Read the model definition and answer for the solid it produces. Units are mm, in the model's axes. A direction names the side the tool comes from. Round coordinates to 2 decimals unless told otherwise and drop trailing zeros. Order: outer loops, then holes, each group sorted by start corner. A loop starts at its lowest first (then second) coordinate and runs counter-clockwise, first axis right, second up. Notation, with made-up numbers: (-38, 1) - (-4, 1) arc R3 cw to (-4, 5) - close; hole circle Ø2 at (50.5, 24.25). An arc over 180 degrees is marked (long way). One line per question, with ' | ' between items. Start each with the question number.
1) Flat-ended cylindrical pins translate along their axes: pin 1 (2 mm diameter, centred on x = 90, z = 0, fed in from -Y); pin 2 (2 mm diameter, centred on y = 15, z = 0, fed in from +X); pin 3 (1.8 mm diameter, centred on x = -150, z = 0, fed in from +Y); pin 4 (11 mm diameter, centred on x = 59, y = 25, fed in from +Z). Find the tip coordinate at first contact, or state that the pin passes through.
2) The mould has two halves that part along Y. Classify faces 3 (the flat face through (-2, 1, -3)), 4 (the flat face through (75.622, -20.278, 1.521)), 5 (the flat face through (-2, 61.188, 0)): pulls with the +Y half, pulls with the -Y half, needs draft (parallel to the pull), parting line crosses it, or undercut.
3) For faces 1 (the flat face through (-2, -61.188, 0)), 2 (the flat face through (63.8, -22.9, 1.5)), determine the directions among +Z, -Z, +X, -X, +Y, -Y from which every point of the face is accessible in a straight line to the end or side of a thin tool.
4) The part is cut by section A-A, the plane y = -34. Give the vertices of the cut face in (x, z).
5) Straight lines are drawn through the part: line 1 (Y direction, x = -146.05, z = 0); line 2 (Z direction, x = -120, y = -57); line 3 (Y direction, x = 104, z = 0.2). For each, find the intervals that lie inside material, in ascending order. Write a range as from..to.
from build123d import *

# Parameters (mm, degrees)
SKETCH_1_W                     = 306
SKETCH_1_H                     = 122.375397488
EXTRUDE_1_DEPTH                = 3
M3X0_5_2_D                     = 2.5
M3X0_5_2_DEPTH                 = 8.5
M3X0_5_2_CBORE_D               = 3
M3X0_5_2_CBORE_DEPTH           = 6
M3X0_5_2_TIP                   = 0.751075774
M3X0_5_2_ON_FACE_2_D           = 2.5
M3X0_5_2_ON_FACE_2_DEPTH       = 8.5
M3X0_5_2_ON_FACE_2_CBORE_D     = 3
M3X0_5_2_ON_FACE_2_CBORE_DEPTH = 6
M3X0_5_2_ON_FACE_2_TIP         = 0.751075774
PATTERN_LINEAR_1_COUNT         = 11
PATTERN_LINEAR_1_PITCH         = 30
CUT_EXTRUDE_1_DEPTH            = 3


# Read off the part's stored shape, not the designer's step: M3x0.5 ねじ穴1
with BuildPart() as part:
    # ｽｹｯﾁ1 → ﾎﾞｽ - 押し出し1 (new, symmetric)
    with BuildSketch(Plane.XY):
        Rectangle(SKETCH_1_W, SKETCH_1_H)
    extrude(amount=EXTRUDE_1_DEPTH, both=True)

    # M3x0.5 ねじ穴1 outline → M3x0.5 ねじ穴1 (revolve, cut)
    with BuildSketch(Plane(origin=(-150, 0, 0), x_dir=(1, 0, 0), z_dir=(0, 0, 1))):
        Polygon((1.25, -52.687698744), (0, -51.93662297), (0, -61.187698744), (1.5, -61.187698744), (1.5, -55.187698744), (1.25, -55.187698744), align=None)
        Polygon((0, 61.187698744), (0, 51.93662297), (1.25, 52.687698744), (1.25, 55.187698744), (1.5, 55.187698744), (1.5, 61.187698744), align=None)
    m3x0_5_1 = revolve(axis=Axis((-150, 0, 0), (0, 1, 0)), mode=Mode.SUBTRACT)

    # M3x0.5 ねじ穴2
    with Locations(Plane(origin=(-153, 45, 0), x_dir=(0, 0, -1), z_dir=(-1, 0, 0))):
        with Locations((0, 0), (0, 30), (0, 60), (0, 90)):
            CounterBoreHole(M3X0_5_2_D / 2, M3X0_5_2_CBORE_D / 2, M3X0_5_2_CBORE_DEPTH, depth=M3X0_5_2_DEPTH)
            with Locations((0, 0, -(M3X0_5_2_DEPTH + M3X0_5_2_TIP / 2))):  # 118° drill point
                Cone(0, M3X0_5_2_D / 2, M3X0_5_2_TIP, mode=Mode.SUBTRACT)

    # M3x0.5 ねじ穴2 on face 2
    with Locations(Plane(origin=(153, -15, 0), x_dir=(0, 0, 1), z_dir=(1, 0, 0))):
        with Locations((0, 0), (0, -30), (0, -60), (0, 30)):
            CounterBoreHole(M3X0_5_2_ON_FACE_2_D / 2, M3X0_5_2_ON_FACE_2_CBORE_D / 2, M3X0_5_2_ON_FACE_2_CBORE_DEPTH, depth=M3X0_5_2_ON_FACE_2_DEPTH)
            with Locations((0, 0, -(M3X0_5_2_ON_FACE_2_DEPTH + M3X0_5_2_ON_FACE_2_TIP / 2))):  # 118° drill point
                Cone(0, M3X0_5_2_ON_FACE_2_D / 2, M3X0_5_2_ON_FACE_2_TIP, mode=Mode.SUBTRACT)

    # 直線ﾊﾟﾀｰﾝ1: M3x0.5 ねじ穴1 ×11
    with Locations(*[(i * PATTERN_LINEAR_1_PITCH, 0, 0) for i in range(1, PATTERN_LINEAR_1_COUNT)]):
        add(m3x0_5_1, mode=Mode.SUBTRACT)

    # ｽｹｯﾁ5 → ｶｯﾄ - 押し出し1 (cut)
    with BuildSketch(Plane.XY.offset(3)):
        Polygon((133, 3), (133, 38.047137303), (19.828606516, 3), align=None)
        Polygon((-3, 41.187698744), (-122.858751899, 41.187698744), (-3, 4.069607278), align=None)
        Polygon((-133, 38.047137303), (-133, 3), (-19.828606516, 3), align=None)
        Polygon((-122.858751899, -41.187698744), (-3, -41.187698744), (-3, -4.069607278), align=None)
        Polygon((133, -38.047137303), (133, -3), (19.828606516, -3), align=None)
        Polygon((122.858751899, 41.187698744), (3, 41.187698744), (3, 4.069607278), align=None)
        Polygon((-133, -3), (-133, -38.047137303), (-19.828606516, -3), align=None)
        Polygon((3, -41.187698744), (122.858751899, -41.187698744), (3, -4.069607278), align=None)
    extrude(amount=-CUT_EXTRUDE_1_DEPTH, mode=Mode.SUBTRACT)


solid = part.part
Values:
1) pin 1: stops at y = -52.54 | pin 2: stops at x = 144.35 | pin 3: stops at y = 52.48 | pin 4: stops at z = 3
2) face 3: needs draft | face 4: undercut | face 5: pulls with the +Y half
3) face 1: +Z, -Z, +X, -X, -Y | face 2: +Z
4) outline: (-153, -3) - (153, -3) - (153, 3) - (133, 3) - (133, 0) - (119.93, 0) - (119.93, 3) - (99.65, 3) - (99.65, 0) - (3, 0) - (3, 3) - (-3, 3) - (-3, 0) - (-99.65, 0) - (-99.65, 3) - (-119.93, 3) - (-119.93, 0) - (-133, 0) - (-133, 3) - (-153, 3) - close
5) line 1: y = -61.19..-46.25, -43.75..-16.25, -13.75..13.75, 16.25..43.75, 46.25..61.19 | line 2: z = -3..-1.5, 1.5..3 | line 3: y = -61.19..-41.19, -35.35..-29.07, -3..3, 29.07..35.35, 41.19..61.19
